Design review of the part built by this model. Coordinates are the model's own, in mm. Round coordinates to 2 decimals unless told otherwise and drop trailing zeros. Order: outer loops, then holes, each group sorted by start corner. A loop starts at its lowest first (then second) coordinate and runs counter-clockwise, first axis right, second up. Notation, with made-up numbers: (74, 40) - (78, 40) arc R9 ccw to (78, 47) - close; hole circle Ø11 at (9, 59). An arc over 180 degrees is marked (long way). Answer as a JSON object with one key per item and string values. Group by question number.
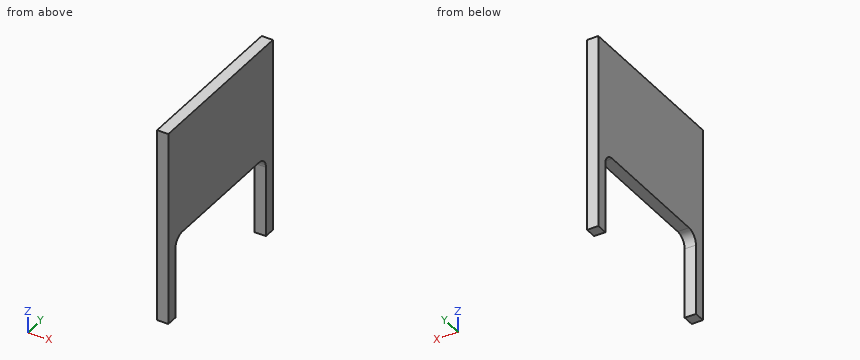
from build123d import *

# Parameters (mm, degrees)
SKETCH1_W           = 219.075
SKETCH1_H           = 190.5
BOSS_EXTRUDE1_DEPTH = 12.7
CUT_EXTRUDE1_REACH  = 147.713
SKETCH2_W           = 92.075
SKETCH2_H           = 165.1
FILLET1_R           = 12.7


with BuildPart() as part:
    # Sketch1 → Boss-Extrude1 (new body)
    with BuildSketch(Plane(origin=(0, 0, 0), x_dir=(0, 0, -1), z_dir=(1, 0, 0))):
        Rectangle(SKETCH1_W, SKETCH1_H)
    extrude(amount=BOSS_EXTRUDE1_DEPTH)

    # Sketch2 → Cut-Extrude1 (cut, up to next)
    with BuildSketch(Plane(origin=(12.7, 0, 0), x_dir=(0, 0, -1), z_dir=(1, 0, 0)), mode=Mode.PRIVATE) as cut_extrude1_sk1:
        with Locations((63.5, 0)):
            Rectangle(SKETCH2_W, SKETCH2_H)
    cut_extrude1_tool1 = extrude(cut_extrude1_sk1.sketch, amount=-CUT_EXTRUDE1_REACH, mode=Mode.PRIVATE) & part.part
    add(cut_extrude1_tool1.solids().sort_by_distance((12.7, 0, -63.5))[0], mode=Mode.SUBTRACT)

    # Fillet1
    fillet1_edges = [part.edges().sort_by_distance(p)[0] for p in [
        (6.35, -82.55, -17.4625),
        (6.35, 82.55, -17.4625),
    ]]
    fillet(fillet1_edges, radius=FILLET1_R)


solid = part.part
1. To check wall thickness, follow line 1 (Y direction, x = 11.75, z = -86); line 2 (Z direction, x = 4.5, y = 44.5); line 3 (Y direction, x = 10.5, z = -19). State the ranges of each line that lie inside material, in increasing order. Write a range as from..to.
2. Take a section at B-B, the plane x = 7.75. Give the boundary of the cut face in (y, z), then the cut area to 3 significant figures.
3. Take a section at C-C, the plane y = -64.5. Give the boundary of the cut face in (x, z), then the cut area to 3 significant figures.
4. Take a section at A-A, the plane z = -38. Give the boundary of the cut face in (x, y), then the cut area to 3 significant figures.
5. Clearance check with a flat-ended pin moving along its axis: P1, Ø1, axis at x = 7, y = 37, coming from the -Z side. State where the tip first meets the part, or that it passes through.
Response values:
{
 "1": {"line 1": "-95.25..-82.55, 82.55..95.25", "line 2": "-17.46..109.54", "line 3": "-95.25..-75.91, 75.91..95.25"},
 "2": {"outline": "(-95.25, -109.54) - (-82.55, -109.54) - (-82.55, -30.16) arc R12.7 cw to (-69.85, -17.46) - (69.85, -17.46) arc R12.7 cw to (82.55, -30.16) - (82.55, -109.54) - (95.25, -109.54) - (95.25, 109.54) - (-95.25, 109.54) - close", "area": "26,600 mm2"},
 "3": {"outline": "(0, -17.46) - (12.7, -17.46) - (12.7, 109.54) - (0, 109.54) - close", "area": "1,610 mm2"},
 "4": {"outline": "(0, -95.25) - (12.7, -95.25) - (12.7, -82.55) - (0, -82.55) - close; (0, 82.55) - (12.7, 82.55) - (12.7, 95.25) - (0, 95.25) - close", "area": "323 mm2"},
 "5": {"P1": "z = -17.46"}
}
